from build123d import *

# Parameters (mm, degrees)
SKETCH_W     = 54
SKETCH_H     = 82
PAD_DEPTH    = 2
SKETCH001_W  = 49
SKETCH001_H  = 77
PAD001_DEPTH = 1
SKETCH002_R  = 3.5
PAD002_DEPTH = 4
SKETCH003_R  = 1.25
POCKET_DEPTH = 7
FILLET_R     = 1
FILLET001_R  = 3


with BuildPart() as part:
    # Sketch → Pad (new body)
    with BuildSketch(Plane.XY):
        Rectangle(SKETCH_W, SKETCH_H)
    extrude(amount=PAD_DEPTH)

    # Sketch001 (on Face6 of Pad) → Pad001 (join)
    with BuildSketch(Plane.XY.offset(2)):
        Rectangle(SKETCH001_W, SKETCH001_H)
    extrude(amount=PAD001_DEPTH)

    # Sketch002 (on Face11 of Pad001) → Pad002 (join)
    with BuildSketch(Plane.XY.offset(3)):
        with Locations((-20.32, 34.29)):
            Circle(SKETCH002_R)
        with Locations((20.32, 34.29)):
            Circle(SKETCH002_R)
        with Locations((-20.32, -34.29)):
            Circle(SKETCH002_R)
        with Locations((20.32, -34.29)):
            Circle(SKETCH002_R)
    extrude(amount=PAD002_DEPTH)

    # Sketch003 (on Face18 of Pad002) → Pocket (cut)
    with BuildSketch(Plane.XY.offset(7)):
        with Locations((-20.32, 34.29)):
            Circle(SKETCH003_R)
        with Locations((20.32, 34.29)):
            Circle(SKETCH003_R)
        with Locations((20.32, -34.29)):
            Circle(SKETCH003_R)
        with Locations((-20.32, -34.29)):
            Circle(SKETCH003_R)
    extrude(amount=-POCKET_DEPTH, mode=Mode.SUBTRACT)

    # Fillet
    fillet_edges = [part.edges().sort_by_distance(p)[0] for p in [
        (-27, 0, 0),
        (0, -41, 0),
        (-27, -41, 1),
        (-27, 41, 1),
        (0, 41, 0),
        (27, 41, 1),
        (27, 0, 0),
        (27, -41, 1),
    ]]
    fillet(fillet_edges, radius=FILLET_R)

    # Fillet001
    fillet001_edges = [part.edges().sort_by_distance(p)[0] for p in [
        (24.5, -38.5, 2.5),
        (24.5, 38.5, 2.5),
        (-24.5, 38.5, 2.5),
        (-24.5, -38.5, 2.5),
    ]]
    fillet(fillet001_edges, radius=FILLET001_R)


solid = part.part
CAD build for the part. Positions are in the model's coordinates, mm. A direction names the side the tool comes from. Give positions to 0.01 mm unless a question says otherwise; leave off trailing zeros. Write each loop counter-clockwise with the first axis right and the second up, starting at its lowest first coordinate (ties: lowest second). Pieces come first, ordered by that corner, then holes. Notation, with made-up numbers: M 81,36 L 87,36 A10 ccw 87,50 Z; hole C 71,35.5 d3. An arc over 180 degrees is marked long. Put each result on its own line as item: value. Start each with the question number.
(1) Mould opens along Y. For faces 6 (the face through (17.543, -36.42, 4.972)), 7 (the face through (-23.6, 37.64, 2.51)), 8 (the face through (-20, -36, 7)) say: +Y half, -Y half, draft (parallel to the pull), parting line (faces both ways), or undercut.
(2) Band-saw the part on D-D, the plane x = 2. Write the cut outline in (y, z).
(3) Band-saw the part on A-A, the plane y = -34.29. Write the cut outline in (x, z).
(4) Which spindle directions (+Z, -Z, +X, -X, +Y, -Y) get a long thin tool onto all of the face, cutting with end or side? Do faces 1 (the face through (23.6, -37.64, 2.51)), 2 (the face through (-23.6, -37.64, 2.51)), 3 (the face through (19.07, 34.34, 3.55)), 4 (the face through (0, 1, 3)), 5 (the face through (23.64, 37.6, 2.51)). Say none if no direction does.
(5) Probe L1, parallel to Y at x = 20.32, z = 5; L2, parallel to Z at x = 17, y = -5; L3, parallel to X at y = -31.5, z = 5.25. List the from-to ranges inside material, lowest first.
(6) Flat gauge pins, fed straight in: pin 1 Ø0.5 at (x, z) = (9, 2.5) entering from +Y; pin 2 Ø5 at (x, y) = (-7.5, -17) entering from +Z; pin 3 Ø2 at (x, y) = (-20.32, 34.29) entering from +Z; pin 4 Ø0.5 at (x, z) = (-10.5, 2.5) entering from -Y. Where does each tip first touch, or does it go through?
(7) Band-saw the part on B-B, the plane x = -20.32. Write the cut outline in (y, z).
(8) Band-saw the part on C-C, the plane z = 5.75. Write the cut outline in (x, y).
Response values:
1. face 6: undercut
1. face 7: +Y half
1. face 8: draft
2. outline: M -41,1 A1 ccw -40,0 L 40,0 A1 ccw 41,1 L 41,2 L 38.5,2 L 38.5,3 L -38.5,3 L -38.5,2 L -41,2 Z
3. outline: M -27,1 A1 ccw -26,0 L -21.57,0 L -21.57,7 L -23.82,7 L -23.82,3 L -24.5,3 L -24.5,2 L -27,2 Z; M -19.07,0 L 19.07,0 L 19.07,7 L 16.82,7 L 16.82,3 L -16.82,3 L -16.82,7 L -19.07,7 Z; M 21.57,0 L 26,0 A1 ccw 27,1 L 27,2 L 24.5,2 L 24.5,3 L 23.82,3 L 23.82,7 L 21.57,7 Z
4. face 1: +Z, +X, -Y
4. face 2: +Z, -X, -Y
4. face 3: +Z, -Z
4. face 4: +Z
4. face 5: +Z, +X, +Y
5. L1: y = -37.79 to -35.54, -33.04 to -30.79, 30.79 to 33.04, 35.54 to 37.79
5. L2: z = 0 to 3
5. L3: x = -22.43 to -18.21, 18.21 to 22.43
6. pin 1: stops at y = 38.5
6. pin 2: stops at z = 3
6. pin 3: passes through
6. pin 4: stops at y = -38.5
7. outline: M -41,1 A1 ccw -40,0 L -35.54,0 L -35.54,7 L -37.79,7 L -37.79,3 L -38.5,3 L -38.5,2 L -41,2 Z; M -33.04,0 L 33.04,0 L 33.04,7 L 30.79,7 L 30.79,3 L -30.79,3 L -30.79,7 L -33.04,7 Z; M 35.54,0 L 40,0 A1 ccw 41,1 L 41,2 L 38.5,2 L 38.5,3 L 37.79,3 L 37.79,7 L 35.54,7 Z
8. outline: C -20.32,-34.29 d7; C -20.32,34.29 d7; C 20.32,-34.29 d7; C 20.32,34.29 d7; hole C -20.32,-34.29 d2.5; hole C -20.32,34.29 d2.5; hole C 20.32,-34.29 d2.5; hole C 20.32,34.29 d2.5
